```python
from build123d import *

# Parameters (mm, degrees)
F1_DEPTH = 25


with BuildPart() as f1:
    # F0 (on Front) → F1 (new body, symmetric)
    with BuildSketch(Plane.XZ):
        Polygon((-15.9999988203, -0.8011669839), (-15.9999988203, -15.3011669839), (-3.0999990533, -15.3011669839), (-3.0999990533, -12.3011669839), (-6.0999990533, -12.3011669839), (-6.0999990533, -8.1011669839), (6.1000009467, -8.1011669839), (6.1000009467, -12.3011669839), (3.1000009467, -12.3011669839), (3.1000009467, -15.3011669839), (16.0000009467, -15.3011669839), (16.0000009467, -0.8011669839), (13.0000011797, -0.8011669839), (13.0000011797, 2.1988330161), (16.0000011797, 2.1988330161), (16.0000011797, 16.6988330161), (13.0000011797, 16.6988330161), (1.5, 5.1988330161), (1.5, 2.1988330161), (0, 2.1988330161), (-1.5, 2.1988330161), (-1.5, 5.1988330161), (-12.9999988203, 16.6988330161), (-15.9999988203, 16.6988330161), (-15.9999988203, 2.1988330161), (-12.9999988203, 2.1988330161), (-12.9999988203, -0.8011669839), align=None)
    extrude(amount=F1_DEPTH, both=True)


solid = f1.part
```
Read the model definition and answer for the solid it produces. Units are mm, in the model's axes. A direction names the side the tool comes from. Coordinates: 2 decimals unless noted, no trailing zeros. Write each loop counter-clockwise with the first axis right and the second up, starting at its lowest first coordinate (ties: lowest second). Pieces come first, ordered by that corner, then holes. Notation, with made-up numbers: (20.25, -26.75) -> (42.25, -26.75) arc R12 cw to (42.25, -9.75) -> close; hole circle Ø4 at (64, 71). An arc over 180 degrees is marked (long way). Return JSON: item names as keys, results as strings.
1. A cutting plane is placed at A-A (z = 3.5). Determine the outline of the cut face in (x, y), and give its area (3 significant figures).
Found:
{"outline": "(-16, -25) -> (-1.5, -25) -> (-1.5, 25) -> (-16, 25) -> close; (1.5, -25) -> (16, -25) -> (16, 25) -> (1.5, 25) -> close", "area": "1,450 mm2"}
2. Determine the mould class of faces 5 (the face through (7.3, -0.4, 11)), 6 (the face through (-14, 0, -0.801)), 7 (the face through (16, 0, -8)) for opening direction Z: pulls with the +Z half, pulls with the -Z half, needs draft (parallel to the pull), parting line crosses it, or undercut.
Found:
{"face 5": "pulls with the +Z half", "face 6": "undercut", "face 7": "needs draft"}
3. Each of these flat-tipped pins is pushed along its axis until it touches: P1, Ø0.9, axis at y = -3.5, z = 1, coming from the -X side; P2, Ø2, axis at y = 3, z = 1, coming from the +X side; P3, Ø0.9, axis at x = 0.5, y = 2, coming from the +Z side; P4, Ø1, axis at x = -4, z = 9.5, coming from the +Y side. Where does it stop, or does it pass through?
Found:
{"P1": "x = -13", "P2": "x = 13", "P3": "z = 2.2", "P4": "through"}
4. A cutting plane is placed at C-C (z = 9). Determine the outline of the cut face in (x, y).
Found:
{"outline": "(-16, -25) -> (-5.3, -25) -> (-5.3, 25) -> (-16, 25) -> close; (5.3, -25) -> (16, -25) -> (16, 25) -> (5.3, 25) -> close"}
5. A cutting plane is placed at D-D (x = 11). Determine the outline of the cut face in (y, z), and give its area (3 significant figures).
Found:
{"outline": "(-25, -15.3) -> (25, -15.3) -> (25, 14.7) -> (-25, 14.7) -> close", "area": "1,500 mm2"}
6. Find the intervals of material crossed by line 1 along Z through (x, y) = (-14, -0.5); line 2 along X through (y, z) = (18.5, -13); line 3 along X through (y, z) = (-3.5, -10.5), in increasing order. Write a range as from..to.
Found:
{"line 1": "-15.3..-0.8, 2.2..16.7", "line 2": "-16..-3.1, 3.1..16", "line 3": "-16..-6.1, 6.1..16"}
7. A cutting plane is placed at B-B (y = 8.5). Determine the outline of the cut face in (x, z), and give its area (3 significant figures).
Found:
{"outline": "(-16, -15.3) -> (-3.1, -15.3) -> (-3.1, -12.3) -> (-6.1, -12.3) -> (-6.1, -8.1) -> (6.1, -8.1) -> (6.1, -12.3) -> (3.1, -12.3) -> (3.1, -15.3) -> (16, -15.3) -> (16, -0.8) -> (13, -0.8) -> (13, 2.2) -> (16, 2.2) -> (16, 16.7) -> (13, 16.7) -> (1.5, 5.2) -> (1.5, 2.2) -> (-1.5, 2.2) -> (-1.5, 5.2) -> (-13, 16.7) -> (-16, 16.7) -> (-16, 2.2) -> (-13, 2.2) -> (-13, -0.8) -> (-16, -0.8) -> close", "area": "760 mm2"}
8. A tool of negligible diameter and unlimited length cuts with its end or side. For faces 1 (the face through (-7.2, -0.4, 10.9)), 2 (the face through (5, 0, -12.301)), 3 (the face through (13, 0, 1)), 4 (the face through (3.1, 0, -14)), from which of +Z, -Z, +X, -X, +Y, -Y can it reach the whole face along a straight path? Write none if from no direction.
Found:
{"face 1": "+Z, +Y, -Y", "face 2": "+Y, -Y", "face 3": "+X, +Y, -Y", "face 4": "-Z, +Y, -Y"}
